from build123d import *

# Parameters (mm, degrees)
F0_W      = 25
F0_H      = 11
F1_DEPTH  = 9
F2_W      = 20.6
F2_H      = 10
F3_DEPTH  = 6
F4_W      = 18.6
F4_H      = 10
F5_DEPTH  = 6
F8_R      = 0.5
F11_W     = 40
F11_H     = 6
F11_R     = 2
F12_DEPTH = 3
F13_R     = 1
F14_R     = 2.99999


# Not quite as in the source:
# - a fillet or chamfer is up to 0.001 mm smaller than in the source, because OpenCascade refuses the exact size


with BuildPart() as f1:
    # F0 (on Top) → F1 (new body)
    with BuildSketch(Plane.XY):
        Rectangle(F0_W, F0_H)
    extrude(amount=F1_DEPTH)


with BuildPart() as f3:
    # F2 (on Top) → F3 (new body)
    with BuildSketch(Plane.XY):
        Rectangle(F2_W, F2_H)
    extrude(amount=F3_DEPTH)


with BuildPart() as f5:
    # F4 (on Top) → F5 (new body)
    with BuildSketch(Plane.XY):
        Rectangle(F4_W, F4_H)
    extrude(amount=F5_DEPTH)


with BuildPart() as f5_1:
    # F6: moved
    add(f5.part.moved(Location((0, -5, 0))))


with BuildPart() as f3_1:
    add(f3.part)

    # F7: union F5
    add(f5_1.part)

    # F8
    f8_edges = [f3_1.edges().sort_by_distance(p)[0] for p in [
        (-9.3, -5, 3),
        (9.3, -5, 3),
    ]]
    fillet(f8_edges, radius=F8_R)


with BuildPart() as f3_2:
    # F9: moved
    add(f3_1.part.moved(Location((0, 0.5, 3))))


with BuildPart() as f1_1:
    add(f1.part)

    # F10: cut F3
    add(f3_2.part, mode=Mode.SUBTRACT)

    # F11 (on Top) → F12 (join)
    with BuildSketch(Plane.XY):
        Rectangle(F11_W, F11_H)
        with Locations((-16.5, 0)):
            Circle(F11_R, mode=Mode.SUBTRACT)
        with BuildLine():
            ThreePointArc((18.5, 0), (16.5, -2), (14.5, 0))
            ThreePointArc((14.5, 0), (16.5, 2), (18.5, 0))
        make_face(mode=Mode.SUBTRACT)
    extrude(amount=F12_DEPTH)

    # F13
    f13_edges = [f1_1.edges().sort_by_distance(p)[0] for p in [
        (-12.5, 5.5, 4.5),
        (-12.5, -5.5, 4.5),
        (12.5, -5.5, 4.5),
        (12.5, 5.5, 4.5),
        (12.5, 0, 3),
        (-12.5, 0, 3),
        (-12.5, 0, 9),
        (12.5, 0, 9),
        (-11.4, 5.5, 9),
        (11.4, 5.5, 9),
        (10.9, -5.5, 9),
        (-10.9, -5.5, 9),
    ]]
    fillet(f13_edges, radius=F13_R)

    # F14 (radius 3 in the source; OpenCascade refuses exactly that, so slightly less here)
    f14_edges = [f1_1.edges().sort_by_distance(p)[0] for p in [
        (-20, -3, 1.5),
        (-20, 3, 1.5),
        (20, 3, 1.5),
        (20, -3, 1.5),
    ]]
    fillet(f14_edges, radius=F14_R)


solid = f1_1.part
Read the model definition and answer for the solid it produces. Units are mm, in the model's axes. A direction names the side the tool comes from. Round coordinates to 2 decimals unless told otherwise and drop trailing zeros. Loops run counter-clockwise (first coordinate to the right, second up) from the corner with the lowest first, then second, coordinate; pieces in that order, holes last.
Q1. Which of the six approach directions +Z, -Z, +X, -X, +Y, -Y give full straight-line access (tool end or side, diameter ignored) to faces 4 (the face through (10.3, 0, 6)), 5 (the face through (-18.1, -1.2, 1.5)), 6 (the face through (-10.892, 5.199, 8.715)), 7 (the face through (18.15, 1.38, 3)), 8 (the face through (15, -3, 2))?
Q2. Section B-B on x = 16.5 is taken. Write down the section's boundary in (y, z).
Q3. Determine the mould class of faces 1 (the face through (-10.3, 0, 6)), 2 (the face through (-12.5, 0, 5)), 3 (the face through (-15, 3, 2)) for opening direction X: released by +X, released by -X, zero draft, split by the parting line, or undercut.
Q4. Section A-A on z = 2.25 is taken. Give the number of separate pieces and of enclosed holes in the cut face, and give its area (3 significant figures).
Q5. Section C-C on y = -0.5 is taken. Write down the section's boundary in (x, z).
Q6. Consider probe 1 along Y at (x, z) = (16.5, 0.85); probe 2 along X at (y, z) = (4, 6.5); probe 3 along Z at (x, y) = (-7.5, 4). Determine where each line is inside the solid, lowest interval first.
Q7. Each of these flat-tipped pins is pushed along its axis until it touches: pin 1 (2 mm diameter, centred on x = 15.5, z = 2.5, fed in from +Y); pin 2 (6.5 mm diameter, centred on x = 17.5, y = 1, fed in from +Z); pin 3 (1 mm diameter, centred on y = 2.5, z = 3, fed in from -X); pin 4 (1.5 mm diameter, centred on x = 13.5, z = 7.5, fed in from -Y). Where does it stop, or does it pass through?
Q8. Section D-D on y = -4 is taken. Write down the section's boundary in (x, z), and give its area (3 significant figures).
Output:
1. face 4: +Z, +Y
1. face 5: +Z, -Z
1. face 6: +Z, +X, -X, +Y
1. face 7: +Z, +X, +Y, -Y
1. face 8: +Z, -Z, +X, -Y
2. outline: (-3, 0) - (-2, 0) - (-2, 3) - (-3, 3) - close; (2, 0) - (3, 0) - (3, 3) - (2, 3) - close
3. face 1: undercut
3. face 2: released by -X
3. face 3: zero draft
4. separate pieces: 1
4. enclosed holes: 2
4. area: 331 mm2
5. outline: (-19.96, 0) - (-18.44, 0) - (-18.44, 3) - (-19.96, 3) - close; (-14.56, 0) - (14.56, 0) - (14.56, 3) - (13.5, 3) arc R1 cw to (12.5, 4) - (12.5, 8) arc R1 ccw to (11.5, 9) - (10.3, 9) - (10.3, 3) - (-10.3, 3) - (-10.3, 9) - (-11.5, 9) arc R1 ccw to (-12.5, 8) - (-12.5, 4) arc R1 cw to (-13.5, 3) - (-14.56, 3) - close; (18.44, 0) - (19.96, 0) - (19.96, 3) - (18.44, 3) - close
6. probe 1: y = -3 to -2, 2 to 3
6. probe 2: x = -12.5 to -10.3, 10.3 to 12.5
6. probe 3: z = 0 to 3
7. pin 1: stops at y = 3
7. pin 2: stops at z = 3
7. pin 3: stops at x = -19.24
7. pin 4: passes through
8. outline: (-12.5, 0) - (12.5, 0) - (12.5, 8) arc R1 ccw to (11.5, 9) - (10.3, 9) - (10.3, 3) - (-10.3, 3) - (-10.3, 9) - (-11.5, 9) arc R1 ccw to (-12.5, 8) - close
8. area: 101 mm2
